The model under review builds one solid part; all positions refer to its coordinate system, in mm. Coordinates: 2 decimals unless noted, no trailing zeros. Answer as CSV lines item,"result". Start each with the question number.
from build123d import *

# Parameters (mm, degrees)
SKETCH1_R               = 1.984375
BOSS_EXTRUDE1_DEPTH     = 169.87266
SKETCH2_W               = 35.763807095
SKETCH2_H               = 22.705005105
CUT_EXTRUDE1_DEPTH      = 23.05812
CUT_EXTRUDE2_START      = -169.87266
SKETCH2_2_W             = 35.763807095
SKETCH2_2_H             = 22.705005105
CUT_EXTRUDE2_DEPTH      = 23.05812
FILLET1_R               = 7.62
CUT_EXTRUDE3_DEPTH      = 198.390942599
CUT_EXTRUDE3_DEPTH_BACK = 198.390942599
SKETCH6_R               = 2.1
CUT_EXTRUDE4_DEPTH      = 198.390942599
CUT_EXTRUDE4_DEPTH_BACK = 198.390942599
SKETCH7_W               = 96.266326783
SKETCH7_H               = 154.195082356
SKETCH7_H_2             = 4.765737644
CUT_EXTRUDE5_DEPTH      = 101.887240685
CUT_EXTRUDE5_DEPTH_BACK = 101.887240685
SKETCH8_W               = 55.334278697
SKETCH8_H               = 64.985105724


with BuildPart() as part:
    # Sketch1 → Boss-Extrude1 (new body)
    with BuildSketch(Plane(origin=(0, 0, 0), x_dir=(1, 0, 0), z_dir=(0, 1, 0))):
        with BuildLine():
            Line((-9.955287346, -3.607451573), (-6.769721368, -3.607451573))
            Line((-6.769721368, -3.607451573), (8.985913589, -3.607451573))
            Line((8.985913589, -3.607451573), (12.171479568, -3.607451573))
            add(Edge.make_bspline(
                [(10.60289965, -20.752451573), (11.099968974, -15.730201571), (11.630563617, -10.016003166), (12.113997871, -4.296816952), (12.171479568, -3.607451573)],
                knots=[0.384969626, 0.384969626, 0.384969626, 0.384969626, 0.458108671, 0.468131593, 0.468131593, 0.468131593, 0.468131593], degree=3))
            add(Edge.make_bspline(
                [(1.108096111, -99.873778356), (4.527344744, -73.531764163), (7.9865599, -47.187219652), (10.60289965, -20.752451573)],
                knots=[0, 0, 0, 0, 0.384969626, 0.384969626, 0.384969626, 0.384969626], degree=3))
            add(Edge.make_bspline(
                [(1.108096111, -99.873778356), (-2.311152522, -73.531764163), (-5.770367679, -47.187219652), (-8.386707429, -20.752451573)],
                knots=[0, 0, 0, 0, 0.384969626, 0.384969626, 0.384969626, 0.384969626], degree=3))
            add(Edge.make_bspline(
                [(-8.386707429, -20.752451573), (-8.883776753, -15.730201571), (-9.414371396, -10.016003166), (-9.89780565, -4.296816952), (-9.955287346, -3.607451573)],
                knots=[0.384969626, 0.384969626, 0.384969626, 0.384969626, 0.458108671, 0.468131593, 0.468131593, 0.468131593, 0.468131593], degree=3))
        make_face()
        with Locations(Location((1.108108569, -11.326456678, 0), (0, 0, 270))):
            Circle(SKETCH1_R, mode=Mode.SUBTRACT)
    extrude(amount=BOSS_EXTRUDE1_DEPTH)

    # Sketch2 → Cut-Extrude1 (cut)
    with BuildSketch(Plane(origin=(0, 169.87266, 0), x_dir=(1, 0, 0), z_dir=(0, 1, 0))):
        with Locations((7.926616202, -14.959954125)):
            Rectangle(SKETCH2_W, SKETCH2_H)
    extrude(amount=-CUT_EXTRUDE1_DEPTH, mode=Mode.SUBTRACT)

    # Sketch2<2> → Cut-Extrude2 (cut)
    with BuildSketch(Plane(origin=(0, 169.87266, 0), x_dir=(1, 0, 0), z_dir=(0, 1, 0)).offset(CUT_EXTRUDE2_START)):
        with Locations((7.926616202, -14.959954125)):
            Rectangle(SKETCH2_2_W, SKETCH2_2_H)
    extrude(amount=CUT_EXTRUDE2_DEPTH, mode=Mode.SUBTRACT)

    # Fillet1
    fillet1_edges = [part.edges().sort_by_distance(p)[0] for p in [
        (-7.824155374, 11.52906, 26.312456678),
        (10.040347595, 11.52906, 26.312456678),
        (-9.955287346, 84.93633, 3.607451573),
        (12.171479568, 84.93633, 3.607451573),
        (-7.824155374, 158.3436, 26.312456678),
        (10.040347595, 158.3436, 26.312456678),
    ]]
    fillet(fillet1_edges, radius=FILLET1_R)

    # Sketch6 → Cut-Extrude3 (cut, two sides: drawn at the far end of the back side and taken through both)
    with BuildSketch(Plane.XZ.offset(-CUT_EXTRUDE3_DEPTH_BACK)):
        with Locations(Location((1.108096111, 71.933778356, 0), (0, 0, 270))):
            Circle(SKETCH6_R)
        with Locations(Location((1.108096111, 34.760552137, 0), (0, 0, 270))):
            Circle(SKETCH6_R)
    extrude(amount=CUT_EXTRUDE3_DEPTH + CUT_EXTRUDE3_DEPTH_BACK, mode=Mode.SUBTRACT)

    # Sketch7 → Cut-Extrude4 (cut, two sides: drawn at the far end of the back side and taken through both)
    with BuildSketch(Plane(origin=(0, 0, 0), x_dir=(0, 0, -1), z_dir=(1, 0, 0)).offset(-CUT_EXTRUDE4_DEPTH_BACK)):
        with Locations((-51.740614965, 77.097541178)):
            Rectangle(SKETCH7_W, SKETCH7_H)
        with Locations((-51.740614965, 167.489791178)):
            Rectangle(SKETCH7_W, SKETCH7_H_2)
    extrude(amount=CUT_EXTRUDE4_DEPTH + CUT_EXTRUDE4_DEPTH_BACK, mode=Mode.SUBTRACT)

    # Sketch8 → Cut-Extrude5 (cut, two sides: drawn at the far end of the back side and taken through both)
    with BuildSketch(Plane.XZ.offset(-154.195082356).offset(-CUT_EXTRUDE5_DEPTH_BACK)):
        with Locations((-8.071043379, 71.50500954)):
            Rectangle(SKETCH8_W, SKETCH8_H)
    extrude(amount=CUT_EXTRUDE5_DEPTH + CUT_EXTRUDE5_DEPTH_BACK, mode=Mode.SUBTRACT)


solid = part.part
1) Mouldability with a two-part tool opening along Z and no side actions: class faces 1 (the face through (1, 165.107, 31)), 2 (the face through (1.2, 159.73, 36.86)), 3 (the face through (1, 160, 39.012)) as released by +Z, released by -Z, zero draft, split by the parting line, or undercut.
2) Insertion check: pin 1 Ø1 at (y, z) = (162.5, 29) entering from -X; pin 2 Ø5 at (y, z) = (162.5, 30.5) entering from +X. Each pin has a flat end and moves straight along its axis. Give the tip position at first contact, or say it passes through.
3) Wall thickness on L1, parallel to Z at x = 1, y = 164; L2, parallel to X at y = 163.25, z = 34.25; L3, parallel to X at y = 162.75, z = 33.25: over which ranges is each line inside the solid? List them lowest first. Write a range as [from, to].
Result:
1,face 1,"zero draft"
1,face 2,"undercut"
1,face 3,"released by +Z"
2,pin 1,"x = -5.55"
2,pin 2,"x = 9.13"
3,L1,"[26.31, 32.66], [36.86, 39.01]"
3,L2,"[-6.96, -0.93], [3.15, 9.18]"
3,L3,"[-6.94, -0.35], [2.57, 9.16]"
